Verification items for the finished model (mm, model axes). A direction names the side the tool comes from. Coordinates: 2 decimals unless noted, no trailing zeros. Order: outer loops, then holes, each group sorted by start corner. A loop starts at its lowest first (then second) coordinate and runs counter-clockwise, first axis right, second up. Notation, with made-up numbers: M 81,67.25 L 113,67.25 A19 ccw 113,93.25 Z; hole C 71.5,72 d6. An arc over 180 degrees is marked long. Return JSON: item names as keys, results as strings. Group by question number.
1. Section check B-B, the plane y = 693. Record the cut outline in (x, z), plus the area to 3 significant figures.
2. Section check C-C, the plane z = 710. Record the cut outline in (x, y).
3. Mould release check, pull along Z, two halves, no side actions. Record for faces 6 (the flat face through (-236, 522, 965.2)), 7 (the flat face through (-335, 762, 25)), 8 (the flat face through (898, 539, 920.75)): +Z half, -Z half, draft (parallel to the pull), parting line (faces both ways), or undercut.
4. Material ranges on line 1 along Y through (x, z) = (-284.5, 733.5); line 2 along Y through (x, z) = (-8, 203.5); line 3 along X through (y, z) = (527, 77), recorded low to high.
5. Gauge pin test, flat ends, axial feed: pin 1 (5 mm diameter, centred on x = 82, z = 668.5, fed in from +Y); pin 2 (10 mm diameter, centred on y = 506.5, z = 817, fed in from +X). Record the tip position at first contact, or that the pin passes through.
6. Section check A-A, the plane y = 781. Record the cut outline in (x, z), plus the area to 3 significant figures.
7. Set-up check for faces 1 (the flat face through (-50.8, 787, 477)), 2 (the flat face through (898, 539, 44.45)), 3 (the flat face through (898, 817.88, 943)), 4 (the flat face through (-609.6, 401, 25)), 5 (the flat face through (919.48, 249, 445)): record each of +Z, -Z, +X, -X, +Y, -Y from which the full face is reachable in a straight line by a thin tool's end or side.
8. Section check D-D, the plane x = -387.5. Record the cut outline in (y, z), plus the area to 3 significant figures.
```python
from build123d import *

# Parameters (mm, degrees)
F0_W           = 1320.8
F0_H           = 1625.6
F0_W_2         = 1219.2
F0_H_2         = 1524
F1_DEPTH       = 50.8
F2_W           = 50.8
F2_H           = 50.8
F3_DEPTH       = 863.6
F4_W           = 1320.8
F4_H           = 1625.6
F4_W_2         = 1219.2
F4_H_2         = 1524
F5_DEPTH       = 50.8
F6_W           = 609.6
F6_H           = 50.8
F7_DEPTH       = 1524
F9_DEPTH       = 965.201
F10_W          = 50.8
F10_H          = 50.8
F11_DEPTH      = 863.6
F12_W          = 558.8
F12_H          = 254
F13_DEPTH      = 914.4
F14_W          = 914.4
F14_H          = 254
F15_DEPTH      = 1625.601
F16_W          = 1625.6
F16_H          = 965.2
F17_DEPTH      = 5.08
F18_W          = 1625.6
F18_H          = 965.2
F19_DEPTH      = 5.08
F20_W          = 1627.432287
F20_H          = 51.704206
F21_DEPTH      = 53.34
F22_W          = 50.8
F22_H          = 965.2
F23_DEPTH      = 914.4
F23_DEPTH_BACK = 665.48
F24_W          = 670.56
F24_H          = 965.2
F25_DEPTH      = 5.08
F26_W          = 670.56
F26_H          = 965.2
F27_DEPTH      = 5.08
F28_W          = 44.45
F28_H          = 44.45
F29_DEPTH      = 549.543908
F30_W          = 670.56
F30_H          = 1035.416092
F31_DEPTH      = 965.201
F32_W          = 670.56
F32_H          = 38.1
F33_DEPTH      = 914.4


with BuildPart() as f1:
    # F0 (on Top) → F1 (new body)
    with BuildSketch(Plane.XY):
        Rectangle(F0_W, F0_H)
        Rectangle(F0_W_2, F0_H_2, mode=Mode.SUBTRACT)
    extrude(amount=F1_DEPTH)

    # F2 (on face) → F3 (join)
    with BuildSketch(Plane.XY.offset(50.8)):
        with Locations((-635, 787.4)):
            Rectangle(F2_W, F2_H)
        with Locations((635, 787.4)):
            Rectangle(F2_W, F2_H)
        with Locations((635, -787.4)):
            Rectangle(F2_W, F2_H)
        with Locations((-635, -787.4)):
            Rectangle(F2_W, F2_H)
    extrude(amount=F3_DEPTH)

    # F4 (on face) → F5 (join)
    with BuildSketch(Plane.XY.offset(914.4)):
        Rectangle(F4_W, F4_H)
        Rectangle(F4_W_2, F4_H_2, mode=Mode.SUBTRACT)
    extrude(amount=F5_DEPTH)

    # F6 (on face) → F7 (join, through all)
    with BuildSketch(Plane.XZ.offset(-762)):
        with Locations((-304.8, 939.8)):
            Rectangle(F6_W, F6_H)
    extrude(amount=F7_DEPTH)

    # F8 (on face) → F9 (cut, through all)
    with BuildSketch(Plane.XY.offset(965.2)):
        Polygon((0, 812.8), (0, 762), (0, -812.8), (660.4, -812.8), (660.4, 812.8), align=None)
    extrude(amount=-F9_DEPTH, mode=Mode.SUBTRACT)

    # F10 (on face) → F11 (join, through all)
    with BuildSketch(Plane.XY.offset(50.8)):
        with Locations((-25.4, 787.4)):
            Rectangle(F10_W, F10_H)
        with Locations((-25.4, -787.4)):
            Rectangle(F10_W, F10_H)
    extrude(amount=F11_DEPTH)

    # F12 (on face) → F13 (join)
    with BuildSketch(Plane.YZ):
        with Locations((533.4, 127)):
            Rectangle(F12_W, F12_H)
    extrude(amount=F13_DEPTH)

    # F14 (on face) → F15 (cut, through all)
    with BuildSketch(Plane(origin=(0, 812.8, 0), x_dir=(-1, 0, 0), z_dir=(0, 1, 0))):
        with Locations((-457.2, 127)):
            Rectangle(F14_W, F14_H)
    extrude(amount=-F15_DEPTH, mode=Mode.SUBTRACT)

    # F16 (on face) → F17 (join)
    with BuildSketch(Plane.YZ):
        with Locations((0, 482.6)):
            Rectangle(F16_W, F16_H)
    extrude(amount=F17_DEPTH)

    # F18 (on face) → F19 (join)
    with BuildSketch(Plane(origin=(-660.4, 0, 0), x_dir=(0, -1, 0), z_dir=(-1, 0, 0))):
        with Locations((0, 482.6)):
            Rectangle(F18_W, F18_H)
    extrude(amount=F19_DEPTH)

    # F20 (on face) → F21 (join)
    with BuildSketch(Plane(origin=(0, 0, 0), x_dir=(0, -1, 0), z_dir=(-1, 0, 0))):
        with Locations((-1.976996, 25.852103)):
            Rectangle(F20_W, F20_H)
    extrude(amount=F21_DEPTH)

    # F22 (on face) → F23 (join, two sides)
    with BuildSketch(Plane.YZ.offset(5.08)) as f23_sk:
        with Locations((242.936092, 482.6)):
            Rectangle(F22_W, F22_H)
    extrude(amount=F23_DEPTH)
    extrude(f23_sk.sketch, amount=-F23_DEPTH_BACK)

    # F24 (on face) → F25 (join)
    with BuildSketch(Plane(origin=(0, 812.8, 0), x_dir=(-1, 0, 0), z_dir=(0, 1, 0))):
        with Locations((330.2, 482.6)):
            Rectangle(F24_W, F24_H)
    extrude(amount=F25_DEPTH)

    # F26 (on face) → F27 (join)
    with BuildSketch(Plane.XZ.offset(812.8)):
        with Locations((-330.2, 482.6)):
            Rectangle(F26_W, F26_H)
    extrude(amount=F27_DEPTH)

    # F28 (on face) → F29 (join, through all)
    with BuildSketch(Plane(origin=(0, 268.336092, 0), x_dir=(-1, 0, 0), z_dir=(0, 1, 0))):
        with Locations((-897.255, 22.225)):
            Rectangle(F28_W, F28_H)
        with Locations((-897.255, 942.975)):
            Rectangle(F28_W, F28_H)
    extrude(amount=F29_DEPTH)

    # F30 (on face) → F31 (cut, through all)
    with BuildSketch(Plane(origin=(0, 0, 0), x_dir=(1, 0, 0), z_dir=(0, 0, -1))):
        with Locations((-330.2, 300.171954)):
            Rectangle(F30_W, F30_H)
    extrude(amount=-F31_DEPTH, mode=Mode.SUBTRACT)

    # F32 (on face) → F33 (join, through all)
    with BuildSketch(Plane(origin=(0, 0, 0), x_dir=(1, 0, 0), z_dir=(0, 0, -1))):
        with Locations((-330.2, -556.9204)):
            Rectangle(F32_W, F32_H)
    extrude(amount=-F33_DEPTH)


solid = f1.part
```
Answers follow:
{
 "1": {"outline": "M -665.48,0 L -609.6,0 L -609.6,50.8 L -660.4,50.8 L -660.4,914.4 L 0,914.4 L 0,51.7 L -53.34,51.7 L -53.34,0 L 5.08,0 L 5.08,965.2 L -665.48,965.2 Z; M 875.03,0 L 919.48,0 L 919.48,44.45 L 875.03,44.45 Z; M 875.03,920.75 L 919.48,920.75 L 919.48,965.2 L 875.03,965.2 Z", "area": "52,600 mm^2"},
 "2": {"outline": "M -665.48,217.54 L 919.48,217.54 L 919.48,268.34 L 5.08,268.34 L 5.08,817.88 L -665.48,817.88 Z; hole M -660.4,268.34 L 0,268.34 L 0,537.87 L -660.4,537.87 Z; hole M -660.4,575.97 L 0,575.97 L 0,762 L -50.8,762 L -50.8,812.8 L -609.6,812.8 L -609.6,762 L -660.4,762 Z"},
 "3": {"face 6": "+Z half", "face 7": "draft", "face 8": "undercut"},
 "4": {"line 1": "217.54 to 268.34, 537.87 to 575.97, 812.8 to 817.88", "line 2": "217.54 to 268.34, 537.87 to 575.97, 762 to 817.88", "line 3": "-665.48 to -660.4, 0 to 5.08"},
 "5": {"pin 1": "y = 268.34", "pin 2": "x = 5.08"},
 "6": {"outline": "M -665.48,0 L 5.08,0 L 5.08,965.2 L -665.48,965.2 Z; M 875.03,0 L 919.48,0 L 919.48,44.45 L 875.03,44.45 Z; M 875.03,920.75 L 919.48,920.75 L 919.48,965.2 L 875.03,965.2 Z; hole M -609.6,50.8 L -53.34,50.8 L -53.34,51.7 L -50.8,51.7 L -50.8,914.4 L -609.6,914.4 Z", "area": "169,000 mm^2"},
 "7": {"face 1": "none", "face 2": "+X, +Y", "face 3": "+Z, -Z, +X, -X, +Y", "face 4": "-Z", "face 5": "+Z, -Z, +X, +Y, -Y"},
 "8": {"outline": "M 217.54,0 L 268.34,0 L 268.34,914.4 L 537.87,914.4 L 537.87,0 L 575.97,0 L 575.97,914.4 L 812.8,914.4 L 812.8,50.8 L 762,50.8 L 762,0 L 817.88,0 L 817.88,965.2 L 217.54,965.2 Z", "area": "119,000 mm^2"}
}
